For this review, take the finished solid that the model builds, in its own axes (mm). Face numbers are marked on the shaded views. A direction names the side the tool comes from. Give positions to 0.01 mm unless a question says otherwise; leave off trailing zeros. Loops run counter-clockwise (first coordinate to the right, second up) from the corner with the lowest first, then second, coordinate; pieces in that order, holes last. Notation, with made-up numbers: (-23, 42.5) - (14, 42.5) arc R23 cw to (14, 57.5) - close; hole circle Ø2 at (31.25, 48). An arc over 180 degrees is marked (long way). Put each result on its own line as item: value.
from build123d import *

# Parameters (mm, degrees)
SKETCH_1_W          = 15
SKETCH_1_H          = 61.71
EXTRUDE_1_DEPTH     = 14
SKETCH_2_W          = 16
SKETCH_2_H          = 15
CUT_EXTRUDE_1_DEPTH = 28
SKETCH_3_W          = 15
SKETCH_3_H          = 11
SKETCH_3_R          = 1.6
EXTRUDE_2_DEPTH     = 8
CUT_EXTRUDE_2_DEPTH = 61
CHAMFER_1_SIZE      = 2
FILLET_1_R          = 2


with BuildPart() as part:
    # 草图1 → 凸台-拉伸1 (new, symmetric)
    with BuildSketch(Plane.XY):
        with Locations((0, 30.855)):
            Rectangle(SKETCH_1_W, SKETCH_1_H)
        with BuildLine():
            Line((0, 58.9727417), (-1.13137085, 57.84137085))
            ThreePointArc((-1.13137085, 57.84137085), (0, 55.11), (1.13137085, 57.84137085))
            Line((1.13137085, 57.84137085), (0, 58.9727417))
        make_face(mode=Mode.SUBTRACT)
    extrude(amount=EXTRUDE_1_DEPTH, both=True)

    # 草图2 → 切除-拉伸1 (cut)
    with BuildSketch(Plane.ZY.offset(7.5)):
        with Locations((0, 54.21)):
            Rectangle(SKETCH_2_W, SKETCH_2_H)
    extrude(amount=-CUT_EXTRUDE_1_DEPTH, mode=Mode.SUBTRACT)

    # 草图3 → 凸台-拉伸2 (add)
    # profile 1 of 2: a face of its own
    with BuildSketch(Plane.XZ):
        with Locations((0, 19.5)):
            Rectangle(SKETCH_3_W, SKETCH_3_H)
        with Locations((0, 20)):
            Circle(SKETCH_3_R, mode=Mode.SUBTRACT)
    # profile 2 of 2: a face of its own
    with BuildSketch(Plane.XZ):
        with Locations((0, -19.5)):
            Rectangle(SKETCH_3_W, SKETCH_3_H)
        with Locations(Location((0, -20, 0), (0, 0, 180))):
            Circle(SKETCH_3_R, mode=Mode.SUBTRACT)
    extrude(amount=-EXTRUDE_2_DEPTH)

    # 草图4 → 切除-拉伸2 (cut)
    with BuildSketch(Plane(origin=(0, 46.71, 0), x_dir=(1, 0, 0), z_dir=(0, 1, 0))):
        with BuildLine():
            Line((4.5, -6), (-4.5, -6))
            ThreePointArc((-4.5, -6), (-5.207106781, -5.707106781), (-5.5, -5))
            Line((-5.5, -5), (-5.5, 5))
            ThreePointArc((-5.5, 5), (-5.207106781, 5.707106781), (-4.5, 6))
            Line((-4.5, 6), (4.5, 6))
            ThreePointArc((4.5, 6), (5.207106781, 5.707106781), (5.5, 5))
            Line((5.5, 5), (5.5, -5))
            ThreePointArc((5.5, -5), (5.207106781, -5.707106781), (4.5, -6))
        make_face()
    extrude(amount=-CUT_EXTRUDE_2_DEPTH, mode=Mode.SUBTRACT)

    # 倒角1
    chamfer_1_edges = [part.edges().sort_by_distance(p)[0] for p in [
        (-7.5, 61.71, -11),
        (7.5, 61.71, -11),
        (-7.5, 61.71, 11),
        (7.5, 61.71, 11),
    ]]
    chamfer(chamfer_1_edges, length=CHAMFER_1_SIZE)

    # 圆角1
    fillet_1_edges = [part.edges().sort_by_distance(p)[0] for p in [
        (7.5, 4, 25),
        (-7.5, 4, 25),
        (7.5, 4, -25),
        (-7.5, 4, -25),
    ]]
    fillet(fillet_1_edges, radius=FILLET_1_R)


solid = part.part
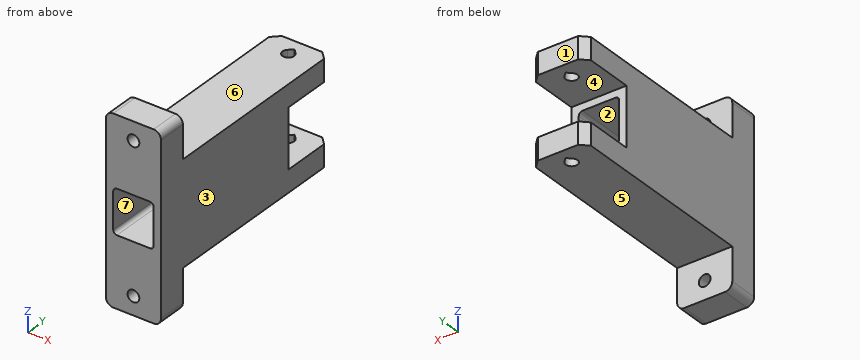
1) Take a section at D-D on x = 6.5. State the section outline as (y, z) points, and give its area (3 significant figures).
Geometry check:
outline: (0, -24.73) - (8, -24.73) - (8, -14) - (60.71, -14) - (60.71, -8) - (46.71, -8) - (46.71, 8) - (60.71, 8) - (60.71, 14) - (8, 14) - (8, 24.73) - (0, 24.73) - close
area: 1,650 mm²
2) Take a section at A-A on z = 20. State the section outline as (x, y) points.
Geometry check:
outline: (-7.5, 0) - (-1.6, 0) - (-1.6, 8) - (-7.5, 8) - close; (1.6, 0) - (7.5, 0) - (7.5, 8) - (1.6, 8) - close
3) Take a section at B-B on y = 56.71. State the section outline as (x, z) points, and give its area (3 significant figures).
Geometry check:
outline: (-7.5, -14) - (-1.6, -14) - (-1.6, -8) - (-7.5, -8) - close; (-7.5, 8) - (-1.6, 8) - (-1.6, 14) - (-7.5, 14) - close; (1.6, -14) - (7.5, -14) - (7.5, -8) - (1.6, -8) - close; (1.6, 8) - (7.5, 8) - (7.5, 14) - (1.6, 14) - close
area: 142 mm²
4) Take a section at C-C on y = 25.5. State the section outline as (x, z) points, and give its area (3 significant figures).
Geometry check:
outline: (-7.5, -14) - (7.5, -14) - (7.5, 14) - (-7.5, 14) - close; hole (-5.5, -5) arc R1 ccw to (-4.5, -6) - (4.5, -6) arc R1 ccw to (5.5, -5) - (5.5, 5) arc R1 ccw to (4.5, 6) - (-4.5, 6) arc R1 ccw to (-5.5, 5) - close
area: 289 mm²
5) Insertion check: pin 1 Ø2.5 at (x, y) = (0, 56.71) entering from +Z; pin 2 Ø8 at (x, y) = (-5.5, 55) entering from -Z; pin 3 Ø4.5 at (x, y) = (2.5, 56) entering from +Z; pin 4 Ø3.5 at (x, z) = (3, -20) entering from +Y. Each pin has a flat end and moves straight along its axis. Give the tip position at first contact, or say it passes through.
Geometry check:
pin 1: passes through
pin 2: stops at z = -14
pin 3: stops at z = 14
pin 4: stops at y = 8
6) Wall thickness on line 1 (Z direction, x = 0, y = 2); line 2 (X direction, y = 33, z = -3); line 3 (X direction, y = 2.25, z = -20): over which ranges is each line inside the solid? List them lowest first.
Geometry check:
line 1: z = -25 to -21.6, -18.4 to -6, 6 to 18.4, 21.6 to 25
line 2: x = -7.5 to -5.5, 5.5 to 7.5
line 3: x = -7.5 to -1.6, 1.6 to 7.5
7) For the marked faces 4, 5, 6 and 7, list the 3-axis set-ups (+Z, -Z, +X, -X, +Y, -Y) from which the entire face can be reached by the end or side of a thin tool; tool diameter is ignored.
Geometry check:
face 4: +X, -X, +Y
face 5: -Z, +X, -X, +Y
face 6: +Z, +X, -X, +Y
face 7: +Y, -Y
8) Draft analysis for pull direction X (two halves, no side actions). For the marked faces 1, 2 and 3, state which applies: pulls with the +X half, pulls with the -X half, needs draft (parallel to the pull), parting line crosses it, or undercut.
Geometry check:
face 1: needs draft
face 2: undercut
face 3: pulls with the +X half
